Work out the finished part from the listing and answer in its coordinate system (mm). Face numbers are marked on the shaded views. A direction names the side the tool comes from. Round coordinates to 2 decimals unless told otherwise and drop trailing zeros. Write each loop counter-clockwise with the first axis right and the second up, starting at its lowest first coordinate (ties: lowest second). Pieces come first, ordered by that corner, then holes. Notation, with made-up numbers: (58.5, -23.75) -> (105.5, -23.75) arc R4 cw to (105.5, -19.75) -> close; hole circle Ø1 at (-31.75, 64). An arc over 180 degrees is marked (long way). One line per question, with ' | ' between items. Start each with the question number.
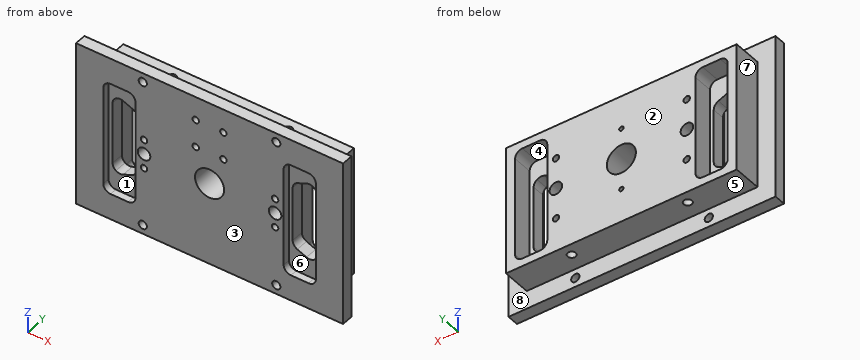
```python
from build123d import *

# Parameters (mm, degrees)
MAIN_SKETCH_W                         = 73.5
MAIN_SKETCH_H                         = 45.5
MAIN_SKETCH_W_2                       = 63.5
MAIN_SKETCH_H_2                       = 35.5
LIP_DEPTH                             = 3.175
MOUNTING_BASE_OUTLINE_W               = 63.5
MOUNTING_BASE_OUTLINE_H               = 35.5
MOUNTING_BASE_OUTLINE_R               = 1.7272
MOUNTING_BASE_OUTLINE_R_2             = 4
MOUNTING_BASE_DEPTH                   = 11
HEATER_CART_4_40_TAPS_D               = 2.2606
HEATER_CART_4_40_TAPS_DEPTH           = 7.595
HEATER_CART_4_40_TAPS_TIP             = 0.679152758
HEATER_CART_4_40_TAPS_ON_FACE_2_D     = 2.2606
HEATER_CART_4_40_TAPS_ON_FACE_2_DEPTH = 7.595
HEATER_CART_4_40_TAPS_ON_FACE_2_TIP   = 0.679152758
MAIN_SKETCH_12_W                      = 8.85
MAIN_SKETCH_12_H                      = 31.2
BOTTOM_SQUARE_CUTOUT_DEPTH            = 2
SQUARE_MICRO_D_CUTOUT_START           = 5.5
SQUARE_MICRO_D_CUTOUT_OUTLINE_W       = 8.85
SQUARE_MICRO_D_CUTOUT_OUTLINE_H       = 31.2
SQUARE_MICRO_D_CUTOUT_DEPTH           = 5.5
MAIN_SKETCH_7_R                       = 0.285
ROUND_MICRO_D_CUTOUT_DEPTH            = 11
INTERNAL_CORNER_CUTOUTS_FILLET_R      = 2
CHIP_CLAMP_0_80_TAPS_AT_2_COUNT       = 2
CHIP_CLAMP_0_80_TAPS_AT_2_PITCH       = 17.1232
CHIP_CLAMP_0_80_TAPS_AT_3_COUNT       = 2
CHIP_CLAMP_0_80_TAPS_AT_3_PITCH       = 17.1232
F_2_56_CLOSE_CLEAR_43_0_089_D         = 2.2606
PCB_2_56_TAPS_D                       = 1.778
PCB_2_56_TAPS_DEPTH                   = 5.734
PCB_2_56_TAPS_TIP                     = 0.53416509
BOTTOM_COVER_2_56_TAPS_D              = 1.778
BOTTOM_COVER_2_56_TAPS_DEPTH          = 5.734
BOTTOM_COVER_2_56_TAPS_TIP            = 0.53416509
F_2_56_TAPPED_HOLE1_D                 = 1.778
F_2_56_TAPPED_HOLE1_DEPTH             = 5.734
F_2_56_TAPPED_HOLE1_TIP               = 0.53416509


# Read off the part's stored shape, not the designer's step: Mounting_Base, Square_Micro_D_Cutout
with BuildPart() as part:
    # Main_Sketch → Lip (new body)
    with BuildSketch(Plane(origin=(0, 0, 0), x_dir=(1, 0, 0), z_dir=(0, 1, 0))):
        with Locations((36.75, -22.75)):
            Rectangle(MAIN_SKETCH_W, MAIN_SKETCH_H)
        with Locations((36.75, -22.75)):
            Rectangle(MAIN_SKETCH_W_2, MAIN_SKETCH_H_2, mode=Mode.SUBTRACT)
    extrude(amount=LIP_DEPTH)

    # Mounting_Base outline → Mounting_Base (add)
    with BuildSketch(Plane(origin=(0, 0, 0), x_dir=(1, 0, 0), z_dir=(0, 1, 0))):
        with Locations((36.75, -22.75)):
            Rectangle(MOUNTING_BASE_OUTLINE_W, MOUNTING_BASE_OUTLINE_H)
        with Locations((18.716, -22.75)):
            Circle(MOUNTING_BASE_OUTLINE_R, mode=Mode.SUBTRACT)
        with Locations((36.75, -22.75)):
            Circle(MOUNTING_BASE_OUTLINE_R_2, mode=Mode.SUBTRACT)
        with Locations((54.784, -22.75)):
            Circle(MOUNTING_BASE_OUTLINE_R, mode=Mode.SUBTRACT)
    extrude(amount=MOUNTING_BASE_DEPTH)

    # Heater_Cart_#4-40_Taps
    with Locations(Plane(origin=(52.725, 7.825, 5), x_dir=(-1, 0, 0), z_dir=(0, 0, -1))):
        with Locations((0, 0), (31.95, 0)):
            Hole(HEATER_CART_4_40_TAPS_D / 2, depth=HEATER_CART_4_40_TAPS_DEPTH)
            with Locations((0, 0, -(HEATER_CART_4_40_TAPS_DEPTH + HEATER_CART_4_40_TAPS_TIP / 2))):  # 118° drill point
                Cone(0, HEATER_CART_4_40_TAPS_D / 2, HEATER_CART_4_40_TAPS_TIP, mode=Mode.SUBTRACT)

    # Heater_Cart_#4-40_Taps on face 2
    with Locations(Plane(origin=(20.775, 7.825, 40.5), x_dir=(1, 0, 0), z_dir=(0, 0, 1))):
        with Locations((0, 0), (31.95, 0)):
            Hole(HEATER_CART_4_40_TAPS_ON_FACE_2_D / 2, depth=HEATER_CART_4_40_TAPS_ON_FACE_2_DEPTH)
            with Locations((0, 0, -(HEATER_CART_4_40_TAPS_ON_FACE_2_DEPTH + HEATER_CART_4_40_TAPS_ON_FACE_2_TIP / 2))):  # 118° drill point
                Cone(0, HEATER_CART_4_40_TAPS_ON_FACE_2_D / 2, HEATER_CART_4_40_TAPS_ON_FACE_2_TIP, mode=Mode.SUBTRACT)

    # Main_Sketch<12> → Bottom_square_cutout (cut)
    with BuildSketch(Plane(origin=(0, 0, 0), x_dir=(1, 0, 0), z_dir=(0, 1, 0))):
        with Locations((11.925, -22.75)):
            Rectangle(MAIN_SKETCH_12_W, MAIN_SKETCH_12_H)
        with BuildLine():
            ThreePointArc((11.521574965, -33.196222286), (10.496212222, -33.351578951), (9.521946869, -32.996175702))
            ThreePointArc((9.521946869, -32.996175702), (8.851632057, -32.244424217), (8.609546604, -31.26675))
            Line((8.609546604, -31.26675), (8.609546604, -14.23325))
            ThreePointArc((8.609546604, -14.23325), (8.851632057, -13.255575783), (9.521946869, -12.503824298))
            ThreePointArc((9.521946869, -12.503824298), (10.496212222, -12.148421049), (11.521574965, -12.303777714))
            Line((11.521574965, -12.303777714), (14.054010046, -13.37581902))
            ThreePointArc((14.054010046, -13.37581902), (14.983840891, -14.148001292), (15.3324534, -15.305291306))
            Line((15.3324534, -15.305291306), (15.3324534, -30.194708694))
            ThreePointArc((15.3324534, -30.194708694), (14.983840891, -31.351998708), (14.054010046, -32.12418098))
            Line((14.054010046, -32.12418098), (11.521574965, -33.196222286))
        make_face(mode=Mode.SUBTRACT)
    bottom_square_cutout = extrude(amount=BOTTOM_SQUARE_CUTOUT_DEPTH, mode=Mode.SUBTRACT)

    # Square_Micro_D_Cutout outline → Square_Micro_D_Cutout (cut)
    with BuildSketch(Plane(origin=(0, 0, 0), x_dir=(1, 0, 0), z_dir=(0, 1, 0)).offset(SQUARE_MICRO_D_CUTOUT_START)):
        with Locations((11.925, -22.75)):
            Rectangle(SQUARE_MICRO_D_CUTOUT_OUTLINE_W, SQUARE_MICRO_D_CUTOUT_OUTLINE_H)
        with BuildLine():
            ThreePointArc((11.521574965, -33.196222286), (9.547492447, -33.013373348), (8.609546604, -31.26675))
            Line((8.609546604, -31.26675), (8.609546604, -14.23325))
            ThreePointArc((8.609546604, -14.23325), (9.547492447, -12.486626652), (11.521574965, -12.303777714))
            Line((11.521574965, -12.303777714), (14.054010046, -13.37581902))
            ThreePointArc((14.054010046, -13.37581902), (14.983840891, -14.148001291), (15.3324534, -15.305291306))
            Line((15.3324534, -15.305291306), (15.3324534, -30.194708694))
            ThreePointArc((15.3324534, -30.194708694), (14.983840891, -31.351998709), (14.054010046, -32.12418098))
            Line((14.054010046, -32.12418098), (11.521574965, -33.196222286))
        make_face(mode=Mode.SUBTRACT)
    square_micro_d_cutout = extrude(amount=SQUARE_MICRO_D_CUTOUT_DEPTH, mode=Mode.SUBTRACT)

    # Main_Sketch<7> → Round_Micro_D_Cutout (cut)
    # profile 1 of 2: a face of its own
    with BuildSketch(Plane(origin=(0, 0, 0), x_dir=(1, 0, 0), z_dir=(0, 1, 0))):
        with BuildLine():
            ThreePointArc((9.521946869, -32.996175702), (8.851632057, -32.244424217), (8.609546604, -31.26675))
            Line((8.609546604, -31.26675), (8.609546604, -14.23325))
            ThreePointArc((8.609546604, -14.23325), (8.851632057, -13.255575783), (9.521946869, -12.503824298))
            ThreePointArc((9.521946869, -12.503824298), (10.496212222, -12.148421049), (11.521574965, -12.303777714))
            Line((11.521574965, -12.303777714), (14.054010046, -13.37581902))
            ThreePointArc((14.054010046, -13.37581902), (14.983840891, -14.148001292), (15.3324534, -15.305291306))
            Line((15.3324534, -15.305291306), (15.3324534, -30.194708694))
            ThreePointArc((15.3324534, -30.194708694), (14.983840891, -31.351998708), (14.054010046, -32.12418098))
            Line((14.054010046, -32.12418098), (11.521574965, -33.196222286))
            ThreePointArc((11.521574965, -33.196222286), (10.496212222, -33.351578951), (9.521946869, -32.996175702))
        make_face()
        with Locations((11.399546604, -22.75)):
            Circle(MAIN_SKETCH_7_R, mode=Mode.SUBTRACT)
    # profile 2 of 2: a face of its own
    with BuildSketch(Plane(origin=(0, 0, 0), x_dir=(1, 0, 0), z_dir=(0, 1, 0))):
        with Locations((11.399546604, -22.75)):
            Circle(MAIN_SKETCH_7_R)
    round_micro_d_cutout = extrude(amount=ROUND_MICRO_D_CUTOUT_DEPTH, mode=Mode.SUBTRACT)

    # MicroD_Mirror: Bottom_square_cutout, Square_Micro_D_Cutout, Round_Micro_D_Cutout across plane
    add(bottom_square_cutout.mirror(Plane(origin=(36.75, 0, 0), x_dir=(0, 0, 1), z_dir=(1, 0, 0))), mode=Mode.SUBTRACT)
    add(square_micro_d_cutout.mirror(Plane(origin=(36.75, 0, 0), x_dir=(0, 0, 1), z_dir=(1, 0, 0))), mode=Mode.SUBTRACT)
    add(round_micro_d_cutout.mirror(Plane(origin=(36.75, 0, 0), x_dir=(0, 0, 1), z_dir=(1, 0, 0))), mode=Mode.SUBTRACT)

    # Internal_Corner_cutouts_fillet
    internal_corner_cutouts_fillet_edges = [part.edges().sort_by_distance(p)[0] for p in [
        (16.35, 8.25, 38.35),
        (7.5, 8.25, 38.35),
        (7.5, 8.25, 7.15),
        (16.35, 8.25, 7.15),
        (57.15, 1, 7.15),
        (57.15, 1, 38.35),
        (66, 1, 38.35),
        (66, 1, 7.15),
        (66, 8.25, 7.15),
        (66, 8.25, 38.35),
        (57.15, 8.25, 38.35),
        (57.15, 8.25, 7.15),
        (16.35, 1, 38.35),
        (16.35, 1, 7.15),
        (7.5, 1, 7.15),
        (7.5, 1, 38.35),
    ]]
    fillet(internal_corner_cutouts_fillet_edges, radius=INTERNAL_CORNER_CUTOUTS_FILLET_R)

    # Sketch3 → Chip_Clamp_#0-80 Taps (revolve, cut)
    with BuildSketch(Plane(origin=(36.75, 11, 31.3116), x_dir=(0, 0, 1), z_dir=(1, 0, 0))):
        Polygon((0, 0), (0, 4.358890611), (0.59563, 4.001), (0.59563, 0), align=None)
    chip_clamp_0_80_taps = revolve(axis=Axis((36.75, 17.35, 31.3116), (0, -1, 0)), mode=Mode.SUBTRACT)

    # Chip_Clamp_#0-80 Taps at 2: Chip_Clamp_#0-80 Taps ×2
    with Locations(*[(0, 0, -i * CHIP_CLAMP_0_80_TAPS_AT_2_PITCH) for i in range(1, CHIP_CLAMP_0_80_TAPS_AT_2_COUNT)]):
        add(chip_clamp_0_80_taps, mode=Mode.SUBTRACT)

    # Chip_Clamp_#0-80 Taps at 3: Chip_Clamp_#0-80 Taps ×2
    with Locations(*[(0, 0, -i * CHIP_CLAMP_0_80_TAPS_AT_3_PITCH) for i in range(1, CHIP_CLAMP_0_80_TAPS_AT_3_COUNT)]):
        add(chip_clamp_0_80_taps, mode=Mode.SUBTRACT)

    # 2-56_Close_Clear#43 (0.089) (through all)
    with Locations(Plane(origin=(18.375, 0, 43), x_dir=(0, 0, -1), z_dir=(0, -1, 0))):
        with Locations((0, 0), (40.5, 0), (40.5, 36.75), (0, 36.75)):
            Hole(F_2_56_CLOSE_CLEAR_43_0_089_D / 2)

    # PCB #2-56 Taps
    with Locations(Plane(origin=(18.75, 11, 14.25), x_dir=(0, 0, 1), z_dir=(0, 1, 0))):
        with Locations((0, 0), (17, 0), (0, 36), (17, 36)):
            Hole(PCB_2_56_TAPS_D / 2, depth=PCB_2_56_TAPS_DEPTH)
            with Locations((0, 0, -(PCB_2_56_TAPS_DEPTH + PCB_2_56_TAPS_TIP / 2))):  # 118° drill point
                Cone(0, PCB_2_56_TAPS_D / 2, PCB_2_56_TAPS_TIP, mode=Mode.SUBTRACT)

    # Bottom_Cover#2-56 Taps
    with Locations(Plane(origin=(54.785, 0, 18.750000125), x_dir=(0, 0, -1), z_dir=(0, -1, 0))):
        with Locations((0, 0), (-8, 0), (-8, -36.07), (0, -36.07)):
            Hole(BOTTOM_COVER_2_56_TAPS_D / 2, depth=BOTTOM_COVER_2_56_TAPS_DEPTH)
            with Locations((0, 0, -(BOTTOM_COVER_2_56_TAPS_DEPTH + BOTTOM_COVER_2_56_TAPS_TIP / 2))):  # 118° drill point
                Cone(0, BOTTOM_COVER_2_56_TAPS_D / 2, BOTTOM_COVER_2_56_TAPS_TIP, mode=Mode.SUBTRACT)

    # #2-56 Tapped Hole1
    with Locations(Plane(origin=(32.94, 0, 31.38), x_dir=(0, 0, -1), z_dir=(0, -1, 0))):
        with Locations((0, 0), (-7.62, 0), (-7.62, 7.62), (0, 7.62)):
            Hole(F_2_56_TAPPED_HOLE1_D / 2, depth=F_2_56_TAPPED_HOLE1_DEPTH)
            with Locations((0, 0, -(F_2_56_TAPPED_HOLE1_DEPTH + F_2_56_TAPPED_HOLE1_TIP / 2))):  # 118° drill point
                Cone(0, F_2_56_TAPPED_HOLE1_D / 2, F_2_56_TAPPED_HOLE1_TIP, mode=Mode.SUBTRACT)


solid = part.part
```
(1) For the marked faces 1, 2, 3, 4 and 5, determine the directions among +Z, -Z, +X, -X, +Y, -Y from which every point of the face is accessible in a straight line to the end or side of a thin tool.
(2) The mould has two halves that part along X. Classify the marked faces 6, 7 and 8: +X half, -X half, draft (parallel to the pull), parting line (faces both ways), or undercut.
(3) Consider L1, parallel to X at y = 5.25, z = 22.75; L2, parallel to Z at x = 18.75, y = 8.4; L3, parallel to X at y = 1, z = 12. Determine where each line is inside the solid, lowest interval first.
(4) A cutting plane is placed at A-A, the plane z = 43. Determine the outline of the cut face in (x, y) (3 decimals).
(5) A cutting plane is placed at B-B, the plane x = 25.5. Determine the outline of the cut face in (y, z) (3 decimals), then the cut area to 3 significant figures.
(6) A cutting plane is placed at C-C, the plane z = 22.75. Count the separate pieces of the cut face and the enclosed holes in it, then the cut area to 3 significant figures.
(7) Given pin 1 Ø1 at (x, y) = (30.5, 9.5) entering from +Z; pin 2 Ø3 at (y, z) = (9.5, 20) entering from -X; pin 3 Ø2 at (x, z) = (55.125, 43) entering from +Y; pin 4 Ø4 at (x, y) = (62, 9.5) entering from -Z, each flat-ended and moving along its own axis, determine where each tip first touches the part or whether it passes through.
Returned:
1) face 1: -Y | face 2: +Z, -Z, +X, -X, +Y | face 3: +Z, -Z, +X, -X, -Y | face 4: +Y | face 5: -Z, +X, -X, +Y
2) face 6: undercut | face 7: -X half | face 8: draft
3) L1: 5 to 8.61, 15.33 to 16.99, 20.44 to 32.75, 40.75 to 53.06, 56.51 to 58.17, 64.89 to 68.5 | L2: 5 to 13.36, 15.14 to 21.02, 24.48 to 30.36, 32.14 to 40.5 | L3: 0 to 7.5, 16.35 to 57.15, 66 to 73.5
4) outline: (0, 0) -> (17.245, 0) -> (17.245, 3.175) -> (0, 3.175) -> close; (19.505, 0) -> (53.995, 0) -> (53.995, 3.175) -> (19.505, 3.175) -> close; (56.255, 0) -> (73.5, 0) -> (73.5, 3.175) -> (56.255, 3.175) -> close
5) outline: (0, 0) -> (3.175, 0) -> (3.175, 5) -> (11, 5) -> (11, 40.5) -> (3.175, 40.5) -> (3.175, 45.5) -> (0, 45.5) -> close | area: 422 mm2
6) separate pieces: 6 | enclosed holes: 0 | area: 386 mm2
7) pin 1: z = 40.5 | pin 2: x = 5 | pin 3: through | pin 4: z = 5
